The listing builds one solid part. Answer for the finished solid, in the listing's coordinates (mm). A direction names the side the tool comes from. Give positions to 0.01 mm unless a question says otherwise; leave off trailing zeros. Order: outer loops, then holes, each group sorted by start corner. A loop starts at its lowest first (then second) coordinate and runs counter-clockwise, first axis right, second up.
```python
from build123d import *

# Parameters (mm, degrees)
SKETCH_1_W               = 10
SKETCH_1_H               = 10
SKETCH_1_W_2             = 8
SKETCH_1_H_2             = 8
EXTRUDE_1_DEPTH          = 70
CUT_EXTRUDE_2_DEPTH      = 71.887234394
CUT_EXTRUDE_2_DEPTH_BACK = 71.887234394
SKETCH_3_R               = 1.6
SKETCH_4_R               = 1.6
CUT_EXTRUDE_3_DEPTH      = 71.887234394


with BuildPart() as part:
    # ｽｹｯﾁ1 → 押し出し-薄板1 (new body)
    with BuildSketch(Plane.XY):
        Rectangle(SKETCH_1_W, SKETCH_1_H)
        Rectangle(SKETCH_1_W_2, SKETCH_1_H_2, mode=Mode.SUBTRACT)
    extrude(amount=EXTRUDE_1_DEPTH)

    # ｽｹｯﾁ3 → ｶｯﾄ - 押し出し2 (cut, two sides: drawn at the far end of the back side and taken through both)
    with BuildSketch(Plane(origin=(0, 5, 0), x_dir=(1, 0, 0), z_dir=(0, 1, 0)).offset(-CUT_EXTRUDE_2_DEPTH_BACK)):
        with Locations(Location((0, -5, 0), (0, 0, 180))):
            Circle(SKETCH_3_R)
        with Locations(Location((0, -15, 0), (0, 0, 180))):
            Circle(SKETCH_3_R)
    extrude(amount=CUT_EXTRUDE_2_DEPTH + CUT_EXTRUDE_2_DEPTH_BACK, mode=Mode.SUBTRACT)

    # ｽｹｯﾁ4 → ｶｯﾄ - 押し出し3 (cut, through all)
    with BuildSketch(Plane.ZY.offset(5)):
        with Locations(Location((67, -2, 0), (0, 0, 270))):
            Circle(SKETCH_4_R)
        with Locations(Location((41.6, -2, 0), (0, 0, 270))):
            Circle(SKETCH_4_R)
    extrude(amount=-CUT_EXTRUDE_3_DEPTH, mode=Mode.SUBTRACT)


solid = part.part
```
1) Straight lines are drawn through the part: probe 1 along Z at (x, y) = (4.4, -2); probe 2 along Z at (x, y) = (0, -4.4); probe 3 along X at (y, z) = (4.45, 5). For each, find the intervals that lie inside material, in ascending order.
Geometry says:
probe 1: z = 0 to 40, 43.2 to 65.4, 68.6 to 70
probe 2: z = 0 to 3.4, 6.6 to 13.4, 16.6 to 70
probe 3: x = -5 to -1.6, 1.6 to 5
2) For a pull along Y with two mould halves and no side action, classify faces 1 (the flat face through (0, -5, 35)), 2 (the cylindrical face through (-4.507, -1.792, 68.586)), 3 (the cylindrical face through (0.208, -4.507, 16.586)), 4 (the flat face through (0, -4, 35)) as +Y half, -Y half, draft (parallel to the pull), parting line (faces both ways), or undercut.
Geometry says:
face 1: -Y half
face 2: undercut
face 3: draft
face 4: undercut
3) Find section C-C (z = 5). Write down the section's boundary in (x, y), then the cut area to 3 significant figures.
Geometry says:
outline: (-5, -5) - (-1.6, -5) - (-1.6, -4) - (-4, -4) - (-4, 4) - (-1.6, 4) - (-1.6, 5) - (-5, 5) - close; (1.6, -5) - (5, -5) - (5, 5) - (1.6, 5) - (1.6, 4) - (4, 4) - (4, -4) - (1.6, -4) - close
area: 29.6 mm2
4) Find section A-A (x = 2.5). Write down the section's boundary in (y, z).
Geometry says:
outline: (-5, 0) - (-4, 0) - (-4, 70) - (-5, 70) - close; (4, 0) - (5, 0) - (5, 70) - (4, 70) - close
5) A tool of negligible diameter and unlimited length cuts with its end or side. For faces 5 (the flat face through (-4, 0, 35)), 6 (the flat face through (-4.5, 0.1, 0)), from which of +Z, -Z, +X, -X, +Y, -Y can it reach the whole face along a straight path? Write none if from no direction.
Geometry says:
face 5: +Z, -Z
face 6: -Z, +X, -X, +Y, -Y
6) Find section B-B (x = 0). Write down the section's boundary in (y, z).
Geometry says:
outline: (-5, 0) - (-4, 0) - (-4, 3.4) - (-5, 3.4) - close; (-5, 6.6) - (-4, 6.6) - (-4, 13.4) - (-5, 13.4) - close; (-5, 16.6) - (-4, 16.6) - (-4, 70) - (-5, 70) - close; (4, 0) - (5, 0) - (5, 3.4) - (4, 3.4) - close; (4, 6.6) - (5, 6.6) - (5, 13.4) - (4, 13.4) - close; (4, 16.6) - (5, 16.6) - (5, 70) - (4, 70) - close
